The drawing under review shows one solid part. Ordinate dimensions are in mm from its lowest x, y, z. Round coordinates to 2 decimals unless told otherwise and drop trailing zeros. Order: outer loops, then holes, each group sorted by start corner. A loop starts at its lowest first (then second) coordinate and runs counter-clockwise, first axis right, second up. Notation, with made-up numbers: (19, 6.25) -> (76, 6.25) arc R36 cw to (76, 43.25) -> close; hole circle Ø11 at (52, 66). An arc over 180 degrees is marked (long way). Use a Markdown table: item, result. Add a question column.
1) Consider section A-A (y = 2.85). State the section outline as (x, z) points (1 decimal).
2) Wall thickness on line 1 along Z through (x, y) = (85, 1.25); line 2 along Z through (x, y) = (59.5, 1.55) (1 decimal); line 3 along Z through (x, y) = (152.5, 3.45) (1 decimal): over which ranges is each line inside the solid? List them lowest first. Write a range as [from, to].
3) Clearance check with flat-ended pins moving along their axes: P1, Ø13, axis at x = 190, z = 30, coming from the -Y side; P2, Ø1.5, axis at y = 2, z = 98, coming from the +X side; P3, Ø1, axis at y = 2, z = 44.5, coming from the +X side; P4, Ø3, axis at x = 185, y = 2, coming from the +Z side. State where each tip first meets the part, or that it passes through.
4) Consider section B-B (z = 30). State the section outline as (x, y) points.
5) Consider section C-C (x = 85). State the section outline as (y, z) points.
6) Consider section D-D (z = 113). State the section outline as (x, y) points.
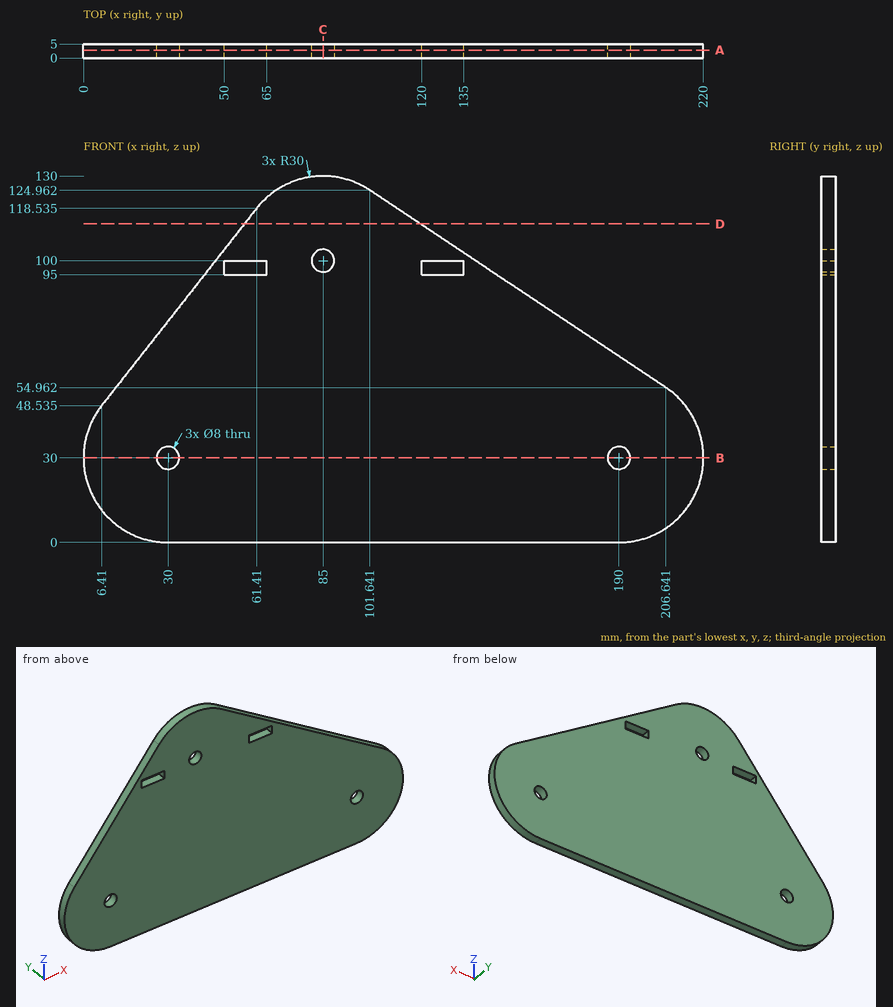
Results list:
| question | item | result |
|---|---|---|
| 1 | outline | (6.4, 48.5) arc R30 ccw to (30, 0) -> (190, 0) arc R30 ccw to (206.6, 55) -> (101.6, 125) arc R30 ccw to (61.4, 118.5) -> close; hole circle Ø8 at (30, 30); hole (50, 95) -> (65, 95) -> (65, 100) -> (50, 100) -> close; hole circle Ø8 at (85, 100); hole (120, 95) -> (135, 95) -> (135, 100) -> (120, 100) -> close; hole circle Ø8 at (190, 30) |
| 2 | line 1 | [0, 96], [104, 130] |
| 2 | line 2 | [0, 95], [100, 116.1] |
| 2 | line 3 | [0, 91.1] |
| 3 | P1 | y = 0 |
| 3 | P2 | x = 143.21 |
| 3 | P3 | x = 216.53 |
| 3 | P4 | z = 70.39 |
| 4 | outline | (0, 0) -> (26, 0) -> (26, 5) -> (0, 5) -> close; (34, 0) -> (186, 0) -> (186, 5) -> (34, 5) -> close; (194, 0) -> (220, 0) -> (220, 5) -> (194, 5) -> close |
| 5 | outline | (0, 0) -> (5, 0) -> (5, 96) -> (0, 96) -> close; (0, 104) -> (5, 104) -> (5, 130) -> (0, 130) -> close |
| 6 | outline | (57.06, 0) -> (119.58, 0) -> (119.58, 5) -> (57.06, 5) -> close |
